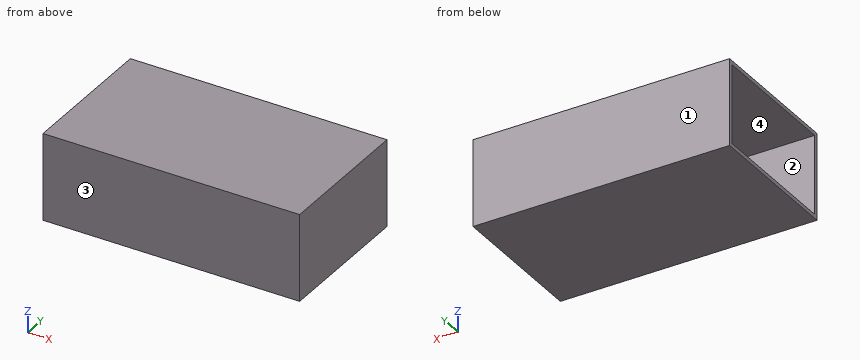
```python
from build123d import *

# Parameters (mm, degrees)
SKETCH1_W           = 670
SKETCH1_H           = 223.333333333
BOSS_EXTRUDE1_DEPTH = 370
SHELL1_T            = -10
SKETCH5_W           = 213.333333333
SKETCH5_H           = 360
CUT_EXTRUDE1_DEPTH  = 10
SKETCH7_W           = 223.333333333
SKETCH7_H           = 370
CUT_EXTRUDE2_DEPTH  = 10


with BuildPart() as part:
    # Sketch1 → Boss-Extrude1 (new body)
    with BuildSketch(Plane(origin=(0, 0, 0), x_dir=(1, 0, 0), z_dir=(0, 1, 0))):
        with Locations((335, 111.666666667)):
            Rectangle(SKETCH1_W, SKETCH1_H)
    extrude(amount=BOSS_EXTRUDE1_DEPTH)

    # Shell1
    shell1_openings = [part.faces().sort_by_distance(p)[0] for p in [
        (0, 185, -111.666666667),
    ]]
    offset(amount=SHELL1_T, openings=shell1_openings, kind=Kind.INTERSECTION)

    # Sketch5 → Cut-Extrude1 (cut)
    with BuildSketch(Plane.ZY):
        with Locations((-111.666666667, 185)):
            Rectangle(SKETCH5_W, SKETCH5_H)
    extrude(amount=-CUT_EXTRUDE1_DEPTH, mode=Mode.SUBTRACT)

    # Sketch7 → Cut-Extrude2 (cut)
    with BuildSketch(Plane.ZY):
        with Locations((-111.666666667, 185)):
            Rectangle(SKETCH7_W, SKETCH7_H)
    extrude(amount=-CUT_EXTRUDE2_DEPTH, mode=Mode.SUBTRACT)


solid = part.part
```
Build history of the part. All positions in model axes, mm. Face numbers are marked on the shaded views. Coordinates: 2 decimals unless noted, no trailing zeros. Order: outer loops, then holes, each group sorted by start corner. A loop starts at its lowest first (then second) coordinate and runs counter-clockwise, first axis right, second up. Notation, with made-up numbers: (19.5, 82.5) -> (68.5, 82.5) arc R21 cw to (68.5, 87.5) -> close; hole circle Ø4 at (55, 80.25). An arc over 180 degrees is marked (long way). Answer in a Markdown table with one row per item. Add a question column.
Q1. Mould opens along Y. For the marked faces 1, 2, 3 and 4 say: +Y half, -Y half, draft (parallel to the pull), parting line (faces both ways), or undercut.
Q2. Band-saw the part on C-C, the plane z = -139.5. List the corners of the cut face in (x, y), then the cut area to 3 significant figures.
Q3. Band-saw the part on A-A, the plane x = 537.5. List the corners of the cut face in (y, z).
Q4. Drop a flat-ended pin along its axis: pin 1 (2 mm diameter, centred on y = 287.5, z = -35.5, fed in from -X). Give the stop position or say it passes through.
Q5. Band-saw the part on B-B, the plane y = 55. List the corners of the cut face in (x, z), then the cut area to 3 significant figures.
Q6. Wall check: line 1 along Z through (x, y) = (57.5, 28.5); line 2 along Y through (x, z) = (358.5, -181.5); line 3 along X through (y, z) = (204, -118.5). Give the ranges that are in metal, low to high. Write a range as [from, to].
Answers follow:
| question | item | result |
|---|---|---|
| 1 | face 1 | +Y half |
| 1 | face 2 | undercut |
| 1 | face 3 | -Y half |
| 1 | face 4 | undercut |
| 2 | outline | (10, 0) -> (670, 0) -> (670, 370) -> (10, 370) -> (10, 360) -> (660, 360) -> (660, 10) -> (10, 10) -> close |
| 2 | area | 16,700 mm^2 |
| 3 | outline | (0, -223.33) -> (370, -223.33) -> (370, 0) -> (0, 0) -> close; hole (10, -213.33) -> (360, -213.33) -> (360, -10) -> (10, -10) -> close |
| 4 | pin 1 | x = 660 |
| 5 | outline | (10, -223.33) -> (670, -223.33) -> (670, 0) -> (10, 0) -> (10, -10) -> (660, -10) -> (660, -213.33) -> (10, -213.33) -> close |
| 5 | area | 15,200 mm^2 |
| 6 | line 1 | [-223.33, -213.33], [-10, 0] |
| 6 | line 2 | [0, 10], [360, 370] |
| 6 | line 3 | [660, 670] |
